```python
from build123d import *

# Parameters (mm, degrees)
SKETCH2_R               = 10
BOSS_EXTRUDE1_DEPTH     = 65
BOSS_EXTRUDE2_DEPTH     = 10
BOSS_EXTRUDE3_DEPTH     = 65
FILLET1_R               = 10
SKETCH5_R               = 4.05
CUT_EXTRUDE1_DEPTH      = 78.781745931
BOSS_EXTRUDE4_DEPTH     = 65
SKETCH8_R               = 4.05
CUT_EXTRUDE3_DEPTH      = 50
CUT_EXTRUDE5_DEPTH      = 92.923881554
CUT_EXTRUDE6_REACH      = 126.298
CUT_EXTRUDE6_END_RADIUS = 17.5
SKETCH7_W               = 12
SKETCH7_H               = 29
CHAMFER1_SIZE           = 13
CHAMFER1_SIZE2          = 35.717206453
FILLET2_R               = 2
SKETCH14_R              = 1.5
CUT_EXTRUDE7_DEPTH      = 100.247166206


with BuildPart() as part:
    # Sketch2 → Boss-Extrude1 (new body)
    with BuildSketch(Plane(origin=(0, 0, 0), x_dir=(1, 0, 0), z_dir=(0, 1, 0))):
        with Locations(Location((0, 0, 0), (0, 0, 270))):
            Circle(SKETCH2_R)
    extrude(amount=-BOSS_EXTRUDE1_DEPTH)

    # Sketch3 → Boss-Extrude2 (add)
    with BuildSketch(Plane(origin=(0, 0, 0), x_dir=(1, 0, 0), z_dir=(0, 1, 0))):
        with BuildLine():
            Line((-10, 0), (-10, -40))
            Line((-10, -40), (15, -40))
            Line((15, -40), (15, 10))
            Line((15, 10), (0, 10))
            ThreePointArc((0, 10), (-7.071067812, 7.071067812), (-10, 0))
        make_face()
    extrude(amount=-BOSS_EXTRUDE2_DEPTH)

    # Sketch4 → Boss-Extrude3 (add)
    with BuildSketch(Plane(origin=(0, 0, 0), x_dir=(1, 0, 0), z_dir=(0, 1, 0))):
        with BuildLine():
            Line((15, 10), (0, 10))
            ThreePointArc((0, 10), (10, 0), (0, -10))
            Line((0, -10), (15, -10))
            Line((15, -10), (15, 10))
        make_face()
    extrude(amount=-BOSS_EXTRUDE3_DEPTH)

    # Fillet1
    fillet1_edges = [part.edges().sort_by_distance(p)[0] for p in [
        (-10, -5, 40),
    ]]
    fillet(fillet1_edges, radius=FILLET1_R)

    # Sketch5 → Cut-Extrude1 (cut, through all)
    with BuildSketch(Plane(origin=(0, 0, 0), x_dir=(1, 0, 0), z_dir=(0, 1, 0))):
        with Locations(Location((0, -31.15, 0), (0, 0, 270))):
            Circle(SKETCH5_R)
        with Locations(Location((0, 0, 0), (0, 0, 270))):
            Circle(SKETCH5_R)
    extrude(amount=-CUT_EXTRUDE1_DEPTH, mode=Mode.SUBTRACT)

    # Sketch6 → Boss-Extrude4 (add)
    with BuildSketch(Plane(origin=(0, 0, 0), x_dir=(1, 0, 0), z_dir=(0, 1, 0))):
        Polygon((15, -40), (35, -40), (35, 60), (15, 60), (15, 10), align=None)
    extrude(amount=-BOSS_EXTRUDE4_DEPTH)

    # Sketch8 → Cut-Extrude3 (cut)
    with BuildSketch(Plane.XY.offset(40)):
        with Locations((25, -7.5)):
            Circle(SKETCH8_R)
        with Locations((25, -57.5)):
            Circle(SKETCH8_R)
    extrude(amount=-CUT_EXTRUDE3_DEPTH, mode=Mode.SUBTRACT)

    # Sketch13 → Cut-Extrude5 (cut, through all)
    with BuildSketch(Plane.ZY.offset(-15)):
        with BuildLine():
            Line((-44.797958971, -18), (-25.202041029, -18))
            ThreePointArc((-25.202041029, -18), (-17.5, -32.5), (-25.202041029, -47))
            Line((-25.202041029, -47), (-44.797958971, -47))
            ThreePointArc((-44.797958971, -47), (-52.5, -32.5), (-44.797958971, -18))
        make_face()
    extrude(amount=-CUT_EXTRUDE5_DEPTH, mode=Mode.SUBTRACT)

    # Cut-Extrude6: up to this cylinder (the profile starts outside it)
    cut_extrude6_end = Plane(origin=(25, -32.5, -35), z_dir=(-1, 0, 0)) * Cylinder(CUT_EXTRUDE6_END_RADIUS, 288.596, mode=Mode.PRIVATE)
    # Sketch7 → Cut-Extrude6 (cut, up to the surface)
    with BuildSketch(Plane.XY.offset(40), mode=Mode.PRIVATE) as cut_extrude6_sk1:
        with Locations((25, -32.5)):
            Rectangle(SKETCH7_W, SKETCH7_H)
    cut_extrude6_tool1 = extrude(cut_extrude6_sk1.sketch, amount=-CUT_EXTRUDE6_REACH, mode=Mode.PRIVATE) - cut_extrude6_end
    add(cut_extrude6_tool1.solids().sort_by_distance((25, -32.5, 40))[0], mode=Mode.SUBTRACT)

    # Chamfer1
    chamfer1_edges = [part.edges().sort_by_distance(p)[0] for p in [
        (25, 0, -60),
        (25, -65, -60),
    ]]
    chamfer1_side = [part.faces().sort_by_distance(p)[0] for p in [
        (25, -32.5, -60),
    ]]
    chamfer(chamfer1_edges, length=CHAMFER1_SIZE, length2=CHAMFER1_SIZE2, reference=chamfer1_side[0])

    # Fillet2
    fillet2_edges = [part.edges().sort_by_distance(p)[0] for p in [
        (7.5, 0, -10),
        (-10, 0, 15),
        (35, -65, 7.858603226),
        (25, -65, -24.282793547),
        (25, -13, -60),
        (25, -52, -60),
        (15, 0, -17.141396774),
        (-7.071067812, 0, -7.071067812),
        (-10, -65, 0),
        (7.5, -65, -10),
        (7.5, -65, 10),
        (17.5, 0, 40),
        (-7.071067812, 0, 37.071067812),
        (15, -37.5, 40),
        (35, -32.5, 40),
        (35, 0, 7.858603226),
        (15, -65, 25),
        (15, -65, -17.141396774),
        (25, -65, 40),
    ]]
    fillet(fillet2_edges, radius=FILLET2_R)

    # Sketch14 → Cut-Extrude7 (cut, through all)
    with BuildSketch(Plane(origin=(35, 0, 0), x_dir=(0, 0, -1), z_dir=(1, 0, 0))):
        with Locations((19.5, -17)):
            Circle(SKETCH14_R)
        with Locations((50.5, -17)):
            Circle(SKETCH14_R)
        with Locations((50.5, -48)):
            Circle(SKETCH14_R)
        with Locations((19.5, -48)):
            Circle(SKETCH14_R)
    extrude(amount=-CUT_EXTRUDE7_DEPTH, mode=Mode.SUBTRACT)


solid = part.part
```
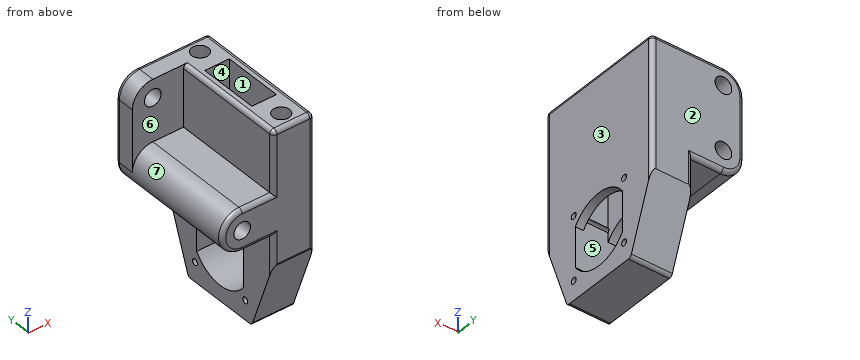
Verification items for the finished model (mm, model axes). Face numbers are marked on the shaded views. A direction names the side the tool comes from. Coordinates: 2 decimals unless noted, no trailing zeros. Write each loop counter-clockwise with the first axis right and the second up, starting at its lowest first coordinate (ties: lowest second). Pieces come first, ordered by that corner, then holes. Notation, with made-up numbers: M 51.5,13.25 L 79.5,13.25 A23 ccw 79.5,33.25 Z; hole C 20.5,35.5 d2. An arc over 180 degrees is marked long. Answer as a JSON object with one key per item and string values. Group by question number.
(1) Tool access check on the marked faces 5, 6 and 7. Record the directions out of +Z, -Z, +X, -X, +Y, -Y that give a thin tool (end or side, any length) a straight path to the whole face; none if there is none.
(2) Material ranges on line 1 (X direction, y = -27, z = 0); line 2 (X direction, y = -36, z = 2); line 3 (Z direction, x = 7, y = -62), recorded low to high.
(3) Cross-section at C-C, the plane z = 17.5. Record the cut outline in (x, y), and give its area (3 significant figures).
(4) Cross-section at A-A, the plane x = 25. State how many separate pieces and enclosed holes the cut face has, and give its area (3 significant figures).
(5) Cross-section at B-B, the plane y = -30.5. Record the cut outline in (x, z), and give its area (3 significant figures).
(6) Cross-section at D-D, the plane z = -50.5. Record the cut outline in (x, y).
(7) Release check for a two-part mould opening along X. For the marked faces 1, 2, 3 and 4 record: +X half, -X half, draft (parallel to the pull), parting line (faces both ways), or undercut.
(8) Gauge pin test, flat ends, axial feed: pin 1 (5 mm diameter, centred on y = -17, z = -50.5, fed in from -X); pin 2 (1.8 mm diameter, centred on y = -48, z = -50.5, fed in from -X); pin 3 (4 mm diameter, centred on x = 26, y = -58.5, fed in from +Z); pin 4 (12 mm diameter, centred on x = 4.5, y = -39, fed in from +Z). Record the tip position at first contact, or that the pin passes through.
Reply:
{
 "1": {"face 5": "none", "face 6": "+Z, -X, -Y", "face 7": "-X, -Y"},
 "2": {"line 1": "-10 to -4.05, 4.05 to 19, 31 to 35", "line 2": "-9.8 to -3.52, 3.52 to 19, 31 to 35", "line 3": "-10 to 10"},
 "3": {"outline": "M -10,-10 L 15,-10 L 15,-63 A2 ccw 17,-65 L 33,-65 A2 ccw 35,-63 L 35,-2 A2 ccw 33,0 L -8,0 A2 ccw -10,-2 Z; hole M 19,-47 L 31,-47 L 31,-18 L 19,-18 Z; hole C 25,-57.5 d8.1; hole C 25,-7.5 d8.1", "area": "1,100 mm²"},
 "4": {"separate pieces": "1", "enclosed holes": "2", "area": "2,580 mm²"},
 "5": {"outline": "M 0,-10 L 15,-10 L 15,-17.61 L 19,-17.61 L 19,40 L 17,40 A2 ccw 15,38 L 15,10 L 0,10 A10 ccw Z; M 15,-60 L 35,-60 L 35,-52.39 L 15,-52.39 Z; M 31,-17.61 L 35,-17.61 L 35,38 A2 ccw 33,40 L 31,40 Z; hole C 0,0 d8.1", "area": "1,020 mm²"},
 "6": {"outline": "M 15,-55.46 L 35,-55.46 L 35,-49.5 L 15,-49.5 Z; M 15,-46.5 L 35,-46.5 L 35,-40.62 L 15,-40.62 Z; M 15,-24.38 L 35,-24.38 L 35,-18.5 L 15,-18.5 Z; M 15,-15.5 L 35,-15.5 L 35,-9.54 L 15,-9.54 Z"},
 "7": {"face 1": "undercut", "face 2": "draft", "face 3": "+X half", "face 4": "undercut"},
 "8": {"pin 1": "x = 15", "pin 2": "through", "pin 3": "z = -10", "pin 4": "z = 10"}
}
